from build123d import *

# Parameters (mm, degrees)
SKETCH1_W                  = 88.9
SKETCH1_H                  = 38.1
BLOCK_DEPTH                = 58.42
SPRING_BORES_D             = 25.4
SPRING_BORES_DEPTH         = 47.625
SPRING_BORES_TIP           = 7.630929862
F_1_2_20_TAPPED_HOLES_D    = 11.50874
VIEW_HOLES_D               = 7.9375
F_10_32_TAPPED_HOLES_D     = 4.0386
F_10_32_TAPPED_HOLES_DEPTH = 19.05
F_10_32_TAPPED_HOLES_TIP   = 1.213317848


with BuildPart() as part:
    # Sketch1 → Block (new body)
    with BuildSketch(Plane(origin=(0, 0, 0), x_dir=(1, 0, 0), z_dir=(0, 1, 0))):
        Rectangle(SKETCH1_W, SKETCH1_H)
    extrude(amount=BLOCK_DEPTH)

    # Spring Bores
    with Locations(Plane(origin=(0, 0, 0), x_dir=(-1, 0, 0), z_dir=(0, -1, 0))):
        with Locations((22.225, 0), (-22.225, 0)):
            Hole(SPRING_BORES_D / 2, depth=SPRING_BORES_DEPTH)
            with Locations((0, 0, -(SPRING_BORES_DEPTH + SPRING_BORES_TIP / 2))):  # 118° drill point
                Cone(0, SPRING_BORES_D / 2, SPRING_BORES_TIP, mode=Mode.SUBTRACT)

    # 1/2-20 Tapped Holes (through all)
    with Locations(Plane(origin=(0, 58.42, 0), x_dir=(1, 0, 0), z_dir=(0, 1, 0))):
        with Locations((-22.225, 0), (22.225, 0)):
            Hole(F_1_2_20_TAPPED_HOLES_D / 2)

    # View Holes (through all)
    with Locations(Plane.XY.offset(19.05)):
        with Locations((-22.225, 47.625), (22.225, 47.625)):
            Hole(VIEW_HOLES_D / 2)

    # #10-32 Tapped Holes
    with Locations(Plane(origin=(0, 0, 0), x_dir=(-1, 0, 0), z_dir=(0, -1, 0))):
        with Locations((0, -11.1125), (0, 11.1125), (36.5125, -11.1125), (36.5125, 11.1125), (-36.5125, 11.1125), (-36.5125, -11.1125)):
            Hole(F_10_32_TAPPED_HOLES_D / 2, depth=F_10_32_TAPPED_HOLES_DEPTH)
            with Locations((0, 0, -(F_10_32_TAPPED_HOLES_DEPTH + F_10_32_TAPPED_HOLES_TIP / 2))):  # 118° drill point
                Cone(0, F_10_32_TAPPED_HOLES_D / 2, F_10_32_TAPPED_HOLES_TIP, mode=Mode.SUBTRACT)


solid = part.part
Build history of the part. All positions in model axes, mm. A direction names the side the tool comes from. Round coordinates to 2 decimals unless told otherwise and drop trailing zeros. Order: outer loops, then holes, each group sorted by start corner. A loop starts at its lowest first (then second) coordinate and runs counter-clockwise, first axis right, second up. Notation, with made-up numbers: M 15,20.25 L 68,20.25 A19 ccw 68,47.25 Z; hole C 83.5,38.25 d3. An arc over 180 degrees is marked long. Use CSV: the item, a comma, the result in double quotes. Start each with the question number.
(1) Flat gauge pins, fed straight in: P1, Ø9, axis at x = 22.225, y = 47.625, coming from the -Z side; P2, Ø3, axis at x = 36.51, z = -11.11, coming from the -Y side; P3, Ø20.5, axis at x = -22.225, z = 0, coming from the -Y side. Where does each tip first touch, or does it go through?
(2) Cut at A-A on z = 0. List the corners of the cut face in (x, y) (3 decimals).
(3) Mould opens along Z. For faces 3 (the face through (36.189, 20.053, 11.247)), 4 (the face through (-44.45, 29, 0)), 5 (the face through (-1, 29, -19.05)) say: +Z half, -Z half, draft (parallel to the pull), parting line (faces both ways), or undercut.
(4) Drill centre lines: probe 1 along X at (y, z) = (37, -10.5); probe 2 along X at (y, z) = (38, 10); probe 3 along Y at (x, z) = (17, 2.5). Where is each one in solid material? Low to high.
(5) Cut at B-B on y = 28.5. List the corners of the cut face in (x, z) (3 decimals).
(6) Cut at C-C on z = 4. State how many separate pieces and enclosed holes the cut face has, then the cut area to 3 significant figures.
(7) Tool access for faces 1 (the face through (-21.71, 51.56, 13.92)), 2 (the face through (33.96, 24.15, 4.86)): list every direction of +Z, -Z, +X, -X, +Y, -Y with a clear straight run to the whole face (end or side of a thin tool).
Findings:
1,P1,"stops at z = -19.05"
1,P2,"stops at y = 19.36"
1,P3,"stops at y = 49.1"
2,outline,"M -44.45,0 L -34.925,0 L -34.925,47.625 L -27.979,51.798 L -27.979,58.42 L -44.45,58.42 Z; M -16.471,51.798 L -9.525,47.625 L -9.525,0 L 9.525,0 L 9.525,47.625 L 16.471,51.798 L 16.471,58.42 L -16.471,58.42 Z; M 27.979,51.798 L 34.925,47.625 L 34.925,0 L 44.45,0 L 44.45,58.42 L 27.979,58.42 Z"
3,face 3,"undercut"
3,face 4,"draft"
3,face 5,"-Z half"
4,probe 1,"x = -44.45 to -29.37, -15.08 to 15.08, 29.37 to 44.45"
4,probe 2,"x = -44.45 to -30.05, -14.4 to 14.4, 30.05 to 44.45"
4,probe 3,"y = 51.78 to 58.42"
5,outline,"M -44.45,-19.05 L 44.45,-19.05 L 44.45,19.05 L -44.45,19.05 Z; hole C -22.225,0 d25.4; hole C 22.225,0 d25.4"
6,separate pieces,"3"
6,enclosed holes,"0"
6,area,"2,650 mm^2"
7,face 1,"+Z, -Z"
7,face 2,"-Y"
